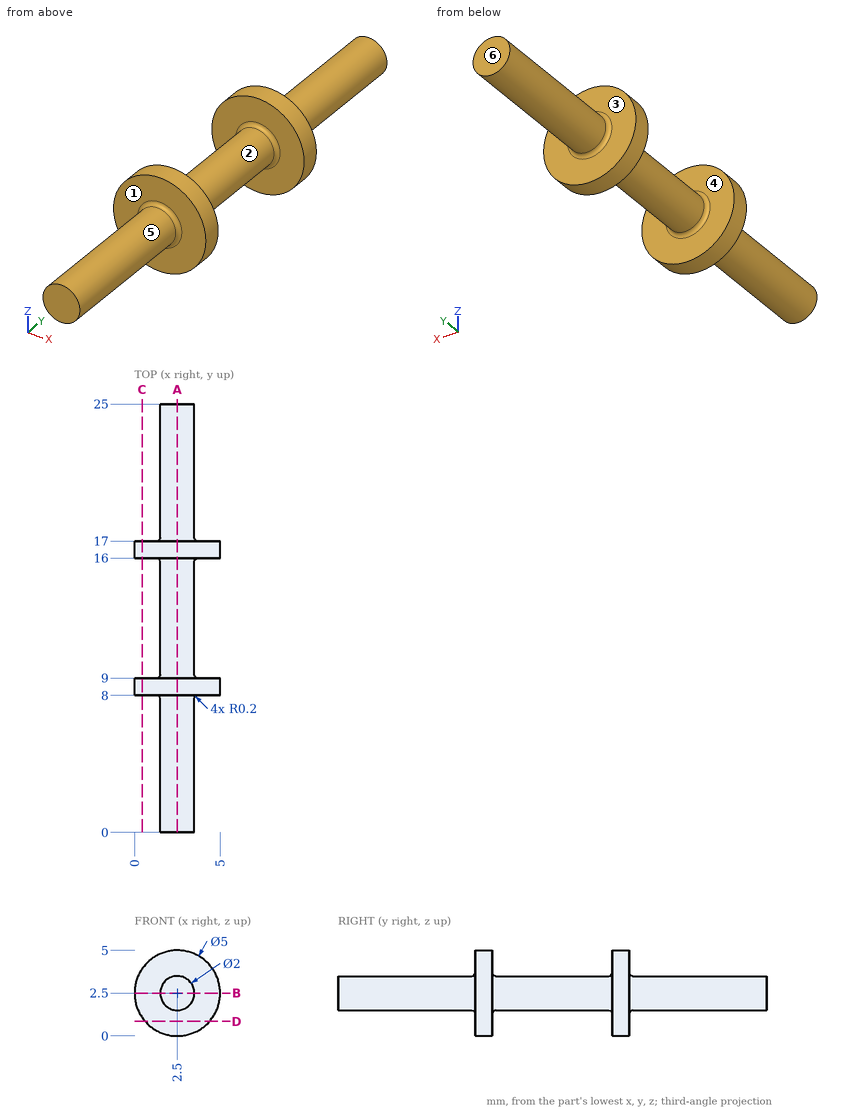
Could you check a few things on this drawing? It's one solid part, dimensions in mm from its lowest x, y, z. A direction names the side the tool comes from. Round coordinates to 2 decimals unless told otherwise and drop trailing zeros. Write each loop counter-clockwise with the first axis right and the second up, starting at its lowest first coordinate (ties: lowest second). Pieces come first, ordered by that corner, then holes. Notation, with made-up numbers: M 62.5,-17.75 L 77.5,-17.75 A8 cw 77.5,-11.75 Z; hole C -2,-18.5 d4. An arc over 180 degrees is marked long. Answer as CSV lines item,"result". Start each with the question number.
1. Suppose I cut it at C-C on x = 0.45. Write out the boundary of the cut face in (y, z), then the cut area to 3 significant figures.
2. I'm going to push flat-ended pins straight in: pin 1 Ø1 at (x, y) = (0.5, 18.5) entering from -Z; pin 2 Ø2 at (y, z) = (22, 3) entering from +X; pin 3 Ø1.5 at (x, z) = (3, 0.5) entering from -Y. Where does each tip first touch, or does it pass through?
3. I need wall thicknesses on probe 1 along Y at (x, z) = (3.45, 4.35); probe 2 along X at (y, z) = (21, 2.25); probe 3 along X at (y, z) = (16.5, 3.5). Which ranges of each line are inside material? Lowest first, please.
4. Suppose I cut it at B-B on z = 2.5. Write out the boundary of the cut face in (x, y).
5. Suppose I cut it at D-D on z = 0.85. Write out the boundary of the cut face in (x, y).
6. Suppose I cut it at A-A on x = 2.5. Write out the boundary of the cut face in (y, z), then the cut area to 3 significant figures.
7. On a 3-axis mill with a long thin cutter (end or side, diameter ignored), from which of +Z, -Z, +X, -X, +Y, -Y can I reach the whole of each face in a straight line? I mean the marked faces 1, 2 and 3. Say none if no direction works.
8. Thinking about a two-plate mould opening in Y: for the marked faces 4, 5 and 6, which applies, released by +Y, released by -Y, zero draft, split by the parting line, or undercut?
Check result:
1,outline,"M 8,1.07 L 9,1.07 L 9,3.93 L 8,3.93 Z; M 16,1.07 L 17,1.07 L 17,3.93 L 16,3.93 Z"
1,area,"5.72 mm2"
2,pin 1,"passes through"
2,pin 2,"stops at x = 3.5"
2,pin 3,"stops at y = 8"
3,probe 1,"y = 8 to 9, 16 to 17"
3,probe 2,"x = 1.53 to 3.47"
3,probe 3,"x = 0.21 to 4.79"
4,outline,"M 0,8 L 1.3,8 A0.2 cw 1.5,7.8 L 1.5,0 L 3.5,0 L 3.5,7.8 A0.2 cw 3.7,8 L 5,8 L 5,9 L 3.7,9 A0.2 cw 3.5,9.2 L 3.5,15.8 A0.2 cw 3.7,16 L 5,16 L 5,17 L 3.7,17 A0.2 cw 3.5,17.2 L 3.5,25 L 1.5,25 L 1.5,17.2 A0.2 cw 1.3,17 L 0,17 L 0,16 L 1.3,16 A0.2 cw 1.5,15.8 L 1.5,9.2 A0.2 cw 1.3,9 L 0,9 Z"
5,outline,"M 0.62,8 L 4.38,8 L 4.38,9 L 0.62,9 Z; M 0.62,16 L 4.38,16 L 4.38,17 L 0.62,17 Z"
6,outline,"M 0,1.5 L 7.8,1.5 A0.2 cw 8,1.3 L 8,0 L 9,0 L 9,1.3 A0.2 cw 9.2,1.5 L 15.8,1.5 A0.2 cw 16,1.3 L 16,0 L 17,0 L 17,1.3 A0.2 cw 17.2,1.5 L 25,1.5 L 25,3.5 L 17.2,3.5 A0.2 cw 17,3.7 L 17,5 L 16,5 L 16,3.7 A0.2 cw 15.8,3.5 L 9.2,3.5 A0.2 cw 9,3.7 L 9,5 L 8,5 L 8,3.7 A0.2 cw 7.8,3.5 L 0,3.5 Z"
6,area,"56.1 mm2"
7,face 1,"-Y"
7,face 2,"none"
7,face 3,"+Y"
8,face 4,"undercut"
8,face 5,"zero draft"
8,face 6,"released by +Y"
